Source: CAD feature listing. Evaluate the final solid. Frame: model axes, mm. A direction names the side the tool comes from. Give positions to 0.01 mm unless a question says otherwise; leave off trailing zeros. Write each loop counter-clockwise with the first axis right and the second up, starting at its lowest first coordinate (ties: lowest second). Pieces come first, ordered by that corner, then holes. Notation, with made-up numbers: M -36,-30.5 L -21,-30.5 A22 cw -21,0.5 Z; hole C 89,-25.75 d9. An arc over 180 degrees is marked long. Return JSON: item names as keys, results as strings.
Autodesk Inventor part; units mm, degrees
ref_plane "YZ Plane" through (0, 0, 0) normal (1, 0, 0) x (0, 1, 0)
ref_plane "XZ Plane" through (0, 0, 0) normal (0, 1, 0) x (-1, 0, 0)
ref_plane "XY Plane" through (0, 0, 0) normal (0, 0, 1) x (1, 0, 0)
sketch "Skizze2" plane through (0, 0, 0) normal (0, 0, 1) x (1, 0, 0)
  line L0 (-36, 116.4167) -> (-56, 116.4167)
  line L1 (-56, 116.4167) -> (-56, 96.4167)
  line L2 (-56, 96.4167) -> (-36, 96.4167)
  line L3 (-36, 96.4167) -> (-36, 116.4167)
  circle A0 centre (-46, 109.75) radius 1.7
  point P0 (0, 0)
  dimension "d0" = 20
  dimension "d1" = 10
  dimension "d2" = 20
  dimension "d3" = 6.6667
extrude "Extrusion1" add sketch "Skizze2" along normal blind 5 contours L3 L2 L1 L0 | A0
sketch "Skizze4" plane through (-56, 96.4167, 0) normal (0, -1, 0) x (1, 0, 0)
  line L0 (0, 0) -> (20, 0)
  line L1 (20, 0) -> (20, 5)
  line L2 (0, 5) -> (20, 5)
  line L3 (0, 0) -> (0, 5)
  line L4 (0, 0) -> (0, 5)
  line L5 (20, 0) -> (20, 5)
  arc A0 (11.927, 22.2993) -> (8.073, 22.2993) centre (10, 20) ccw
  line L6 (10, 20) -> (10, 5) construction
  line L7 (0, 5) -> (20, 5) construction
  arc A1 (8.073, 22.2993) -> (0, 5) centre (22.5714, 5) ccw
  arc A2 (20, 5) -> (11.927, 22.2993) centre (-2.5714, 5) ccw
  circle A3 centre (10, 15) radius 2.65
  point P0 (56, 0)
  dimension "d6" = 6
  dimension "d7" = 15
  dimension "d8" = 23
  dimension "d11" = 5.3
  dimension "d20" = 10
extrude "Extrusion2" add sketch "Skizze4" against normal blind 6.6667 contours A1 A0 A2 L2
sketch "Skizze6" plane through (0, 0, 5) normal (0, 0, 1) x (1, 0, 0)
  circle A0 centre (-46, 109.75) radius 1.7
  point P0 (0, 0)
hole "Bohrung1" at (-46, 109.75, 5) direction (0, 0, -1) diameter 3 end through all countersink diameter 6 countersink angle 90
equation "\"d1\" = 0.5 * d0"
equation "\"d3\" = 0.333333 * d2"
properties part number "Winkel"
1) Draft query along Z for faces 3 (the face through (-46, 107, 0)), 4 (the face through (-48.103, 99.703, 13.388)), 5 (the face through (-46, 100, 23)), 6 (the face through (-36, 106, 2)). Return one class per face: released by +Z, released by -Z, zero draft, split by the parting line, or undercut.
Numbers:
{"face 3": "released by -Z", "face 4": "undercut", "face 5": "released by +Z", "face 6": "zero draft"}
2) Line query: line 1 (X direction, y = 109.75, z = 2.55); line 2 (Z direction, x = -46, y = 101.75); line 3 (Z direction, x = -50.5, y = 111). Output: solid intervals per line, ascending. Write a range as [from, to].
Numbers:
{"line 1": "x = [-56, -47.5], [-44.5, -36]", "line 2": "z = [0, 12.35], [17.65, 23]", "line 3": "z = [0, 5]"}
3) Cut plane B-B, the plane x = -46. Return the cut outline in (y, z), then the cut area to 3 significant figures.
Numbers:
{"outline": "M 96.42,0 L 108.25,0 L 108.25,3.5 L 106.75,5 L 103.08,5 L 103.08,12.35 L 96.42,12.35 Z; M 96.42,17.65 L 103.08,17.65 L 103.08,23 L 96.42,23 Z; M 111.25,0 L 116.42,0 L 116.42,5 L 112.75,5 L 111.25,3.5 Z", "area": "167 mm²"}
4) Cut plane D-D, the plane y = 114.75. Return the cut outline in (x, z), then the cut area to 3 significant figures.
Numbers:
{"outline": "M -56,0 L -36,0 L -36,5 L -56,5 Z", "area": "100 mm²"}
5) Cut plane C-C, the plane z = 15. Return the cut outline in (x, y).
Numbers:
{"outline": "M -53.66,96.42 L -48.65,96.42 L -48.65,103.08 L -53.66,103.08 Z; M -43.35,96.42 L -38.34,96.42 L -38.34,103.08 L -43.35,103.08 Z"}
6) Set-up query: faces 1 (the face through (-46, 113, 5)), 2 (the face through (-45.09, 110.94, 1.73)). Return all of +Z, -Z, +X, -X, +Y, -Y with unobstructed straight access to the full face (end or side cutting, diameter ignored); none if empty.
Numbers:
{"face 1": "+Z, +X, -X, +Y", "face 2": "+Z, -Z"}
7) Contact query for flat-ended pins moving along their axis: pin 1 Ø6 at (x, y) = (-50, 99) entering from -Z; pin 2 Ø3 at (y, z) = (102.5, 20.5) entering from +X; pin 3 Ø5 at (x, y) = (-49, 101.5) entering from +Z; pin 4 Ø3.5 at (x, y) = (-46, 109.75) entering from +Z. Output: stop coordinate, or through.
Numbers:
{"pin 1": "stops at z = 0", "pin 2": "stops at x = -40.87", "pin 3": "stops at z = 22.96", "pin 4": "stops at z = 3.75"}
8) Cut plane A-A, the plane y = 109.75. Return the cut outline in (x, z), then the cut area to 4 significant figures.
Numbers:
{"outline": "M -56,0 L -47.5,0 L -47.5,3.5 L -49,5 L -56,5 Z; M -44.5,0 L -36,0 L -36,5 L -43,5 L -44.5,3.5 Z", "area": "82.75 mm²"}
